Can you work these out from the drawing? Everything is in mm from the part's minimum corner. A direction names the side the tool comes from. Round coordinates to 2 decimals unless told otherwise and drop trailing zeros. Order: outer loops, then holes, each group sorted by start corner. A loop starts at its lowest first (then second) coordinate and runs counter-clockwise, first axis right, second up. Notation, with made-up numbers: (34, 89.25) -> (70, 89.25) arc R18 cw to (70, 106.25) -> close; hole circle Ø4 at (74, 60). An arc over 180 degrees is marked (long way). One line per item, written item: value.
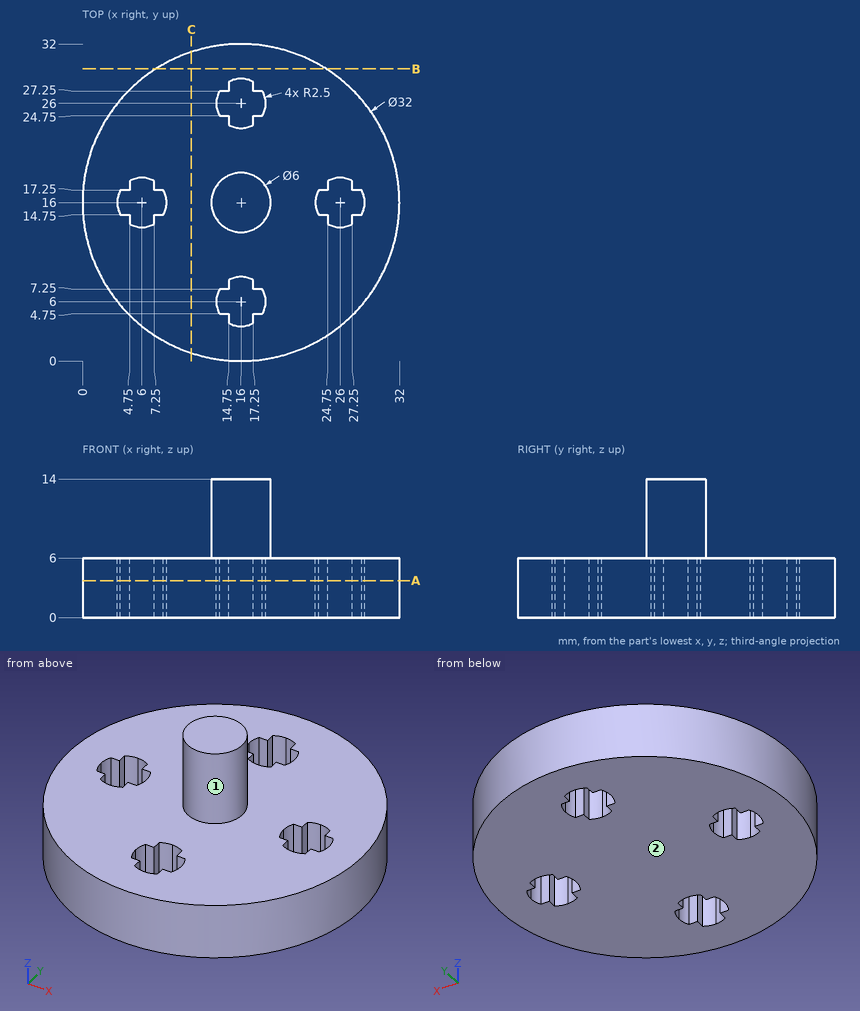
Q1. I need wall thicknesses on line 1 along Y through (x, z) = (16, 2.5); line 2 along Z through (x, y) = (21, 21); line 3 along X through (y, z) = (14, 4.25). Which ranges of each line are inside material? Lowest first, please.
Answers:
line 1: 0 to 3.5, 8.5 to 23.5, 28.5 to 32
line 2: 0 to 6
line 3: 0.13 to 4.75, 7.25 to 24.75, 27.25 to 31.87
Q2. I want a section at A-A on z = 3.75. Give the number of separate pieces and of enclosed holes in the cut face, then the cut area to 3 significant figures.
Answers:
separate pieces: 1
enclosed holes: 4
area: 734 mm2
Q3. I want a section at C-C on x = 11. Write out the boundary of the cut face in (y, z), then the cut area to 3 significant figures.
Answers:
outline: (0.8, 0) -> (31.2, 0) -> (31.2, 6) -> (0.8, 6) -> close
area: 182 mm2
Q4. Which directions (+Z, -Z, +X, -X, +Y, -Y) give clear straight access to the entire face, cutting with the end or side of a thin tool? Please do the marked faces 1 and 2.
Answers:
face 1: +Z
face 2: -Z, +X, -X, +Y, -Y
Q5. For P1, Ø0.7, axis at x = 14, z = 3.5, coming from the -Y side; P2, Ø1.5, axis at x = 27.5, y = 28.5, coming from the -Z side; P3, Ø0.5, axis at y = 24.5, z = 4, coming from the -X side; P4, Ø1, axis at y = 14, z = 3.5, coming from the -X side, each with a flat end and sliding along its axis, tell me the tip position at first contact or that it passes through.
Answers:
P1: y = 0.09
P2: through
P3: x = 2.29
P4: x = 0.07
Q6. I want a section at B-B on y = 29.5. Write out the boundary of the cut face in (x, z), then the cut area to 3 significant figures.
Answers:
outline: (7.41, 0) -> (24.59, 0) -> (24.59, 6) -> (7.41, 6) -> close
area: 103 mm2
